Here's how the part is built. I have some questions about the finished solid (model axes, mm). Give positions to 0.01 mm unless a question says otherwise; leave off trailing zeros. Loops run counter-clockwise (first coordinate to the right, second up) from the corner with the lowest first, then second, coordinate; pieces in that order, holes last. Notation, with made-up numbers: (13, 84) - (60, 84) arc R17 cw to (60, 90) - close; hole circle Ø9 at (27, 42.25). An arc over 180 degrees is marked (long way). Use one line per item in the form item = value.
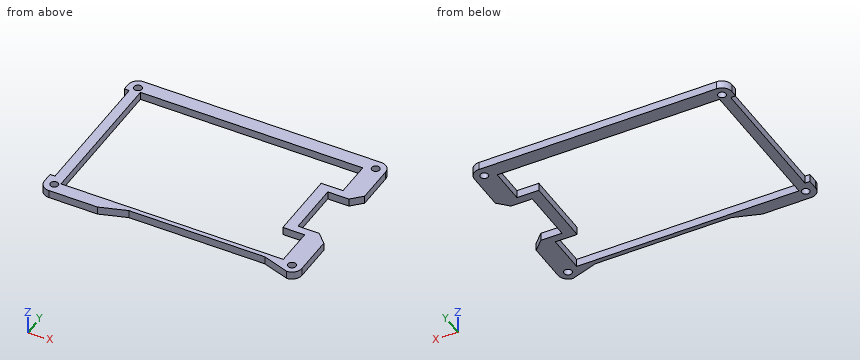
from build123d import *

# Parameters (mm, degrees)
BOSS_EXTRUDE1_DEPTH = 3.048
SKETCH2_R           = 1.355900406
CUT_EXTRUDE1_DEPTH  = 430.898988368
SKETCH3_R           = 1.524
CUT_EXTRUDE2_DEPTH  = 430.898988368
CUT_EXTRUDE3_DEPTH  = 430.898988368
SKETCH4_4_W         = 8.3947
SKETCH4_4_H         = 2.41935
BOSS_EXTRUDE2_DEPTH = 3.048


with BuildPart() as part:
    # Sketch1 → Boss-Extrude1 (new body)
    with BuildSketch(Plane.XY):
        with BuildLine():
            Line((-309.8086, 128.8851), (-305.87795, 128.8851))
            Line((-305.87795, 128.8851), (-301.9473, 132.81575))
            Line((-301.9473, 132.81575), (-301.9473, 150.9704))
            ThreePointArc((-301.9473, 150.9704), (-303.063223164, 153.664476836), (-305.7573, 154.7804))
            Line((-305.7573, 154.7804), (-397.247125, 154.7804))
            ThreePointArc((-397.247125, 154.7804), (-399.946077222, 153.659592612), (-401.0571, 150.956597849))
            Line((-401.0571, 150.956597849), (-401.0571, 148.341))
            Line((-401.0571, 148.341), (-399.1521, 148.341))
            Line((-399.1521, 148.341), (-399.1521, 95.6449))
            Line((-399.1521, 95.6449), (-401.0571, 95.6449))
            Line((-401.0571, 95.6449), (-401.0571, 91.659304166))
            ThreePointArc((-401.0571, 91.659304166), (-399.951018769, 88.947400452), (-397.2472, 87.8217))
            Line((-397.2472, 87.8217), (-378.5565, 87.8217))
            Line((-378.5565, 87.8217), (-368.3165, 91.1883))
            Line((-368.3165, 91.1883), (-315.9973, 91.1883))
            Line((-315.9973, 91.1883), (-305.7573, 87.8217))
            ThreePointArc((-305.7573, 87.8217), (-303.063223164, 88.937623164), (-301.9473, 91.6317))
            Line((-301.9473, 91.6317), (-301.9473, 111.74645))
            Line((-301.9473, 111.74645), (-305.87795, 115.6771))
            Line((-305.87795, 115.6771), (-309.8086, 115.6771))
            Line((-309.8086, 115.6771), (-314.0123, 115.6771))
            Line((-314.0123, 115.6771), (-314.0123, 128.8851))
            Line((-314.0123, 128.8851), (-309.8086, 128.8851))
        make_face()
        Polygon((-395.3675, 92.9525), (-395.3675, 149.2432), (-309.8086, 149.2432), (-309.8086, 132.81575), (-318.2033, 132.81575), (-318.2033, 111.74645), (-309.8086, 111.74645), (-309.8086, 92.9525), align=None, mode=Mode.SUBTRACT)
    extrude(amount=BOSS_EXTRUDE1_DEPTH)

    # Sketch2 → Cut-Extrude1 (cut, through all)
    with BuildSketch(Plane(origin=(0, 0, 0), x_dir=(-1, 0, 0), z_dir=(0, 0, -1))):
        with Locations((305.7573, 150.9704)):
            Circle(SKETCH2_R)
        with Locations((397.247125, 150.9704)):
            Circle(SKETCH2_R)
        with Locations((397.2472, 91.6317)):
            Circle(SKETCH2_R)
        with Locations((305.7573, 91.6317)):
            Circle(SKETCH2_R)
    extrude(amount=-CUT_EXTRUDE1_DEPTH, mode=Mode.SUBTRACT)

    # Sketch3 → Cut-Extrude2 (cut, through all)
    with BuildSketch(Plane(origin=(0, 0, 0), x_dir=(-1, 0, 0), z_dir=(0, 0, -1))):
        with Locations((305.7573, 150.9704)):
            Circle(SKETCH3_R)
        with Locations((397.247125, 150.9704)):
            Circle(SKETCH3_R)
        with Locations((397.2472, 91.6317)):
            Circle(SKETCH3_R)
        with Locations((305.7573, 91.6317)):
            Circle(SKETCH3_R)
    extrude(amount=-CUT_EXTRUDE2_DEPTH, mode=Mode.SUBTRACT)

    # Sketch4 → Cut-Extrude3 (cut, through all)
    with BuildSketch(Plane.XY.offset(3.048)):
        Polygon((-301.9473, 111.74645), (-301.9473, 132.81575), (-305.87795, 128.8851), (-314.0123, 128.8851), (-314.0123, 115.6771), (-305.87795, 115.6771), align=None)
        Polygon((-301.9473, 132.81575), (-301.9473, 136.11775), (-305.87795, 132.1871), (-314.0123, 132.1871), (-314.0123, 128.8851), (-305.87795, 128.8851), align=None)
        Polygon((-301.9473, 107.17445), (-301.9473, 111.74645), (-305.87795, 115.6771), (-314.0123, 115.6771), (-314.0123, 111.74645), (-309.8086, 111.74645), (-309.8086, 111.1051), (-305.87795, 111.1051), align=None)
    extrude(amount=-CUT_EXTRUDE3_DEPTH, mode=Mode.SUBTRACT)

    # Sketch4<4> → Boss-Extrude2 (add)
    with BuildSketch(Plane.XY.offset(3.048)):
        Polygon((-301.9473, 104.12645), (-301.9473, 107.17445), (-305.87795, 111.1051), (-309.8086, 111.1051), (-309.8086, 108.0571), (-305.87795, 108.0571), align=None)
        Polygon((-314.0123, 111.1051), (-314.0123, 111.74645), (-318.2033, 111.74645), (-318.2033, 108.0571), (-309.8086, 108.0571), (-309.8086, 111.1051), align=None)
        with Locations((-314.00595, 134.025425)):
            Rectangle(SKETCH4_4_W, SKETCH4_4_H)
    extrude(amount=-BOSS_EXTRUDE2_DEPTH)


solid = part.part
(1) If we section it at C-C (y = 105): List the corners of the cut face in (x, z) for me, plus the area to 3 significant figures.
Geometry says:
outline = (-399.15, 0) - (-395.37, 0) - (-395.37, 3.05) - (-399.15, 3.05) - close; (-309.81, 0) - (-301.95, 0) - (-301.95, 3.05) - (-309.81, 3.05) - close
area = 35.5 mm²
(2) If I drill on probe 1 along X at (y, z) = (151, 1.5); probe 2 along X at (y, z) = (95, 1.35); probe 3 along Y at (x, z) = (-318.5, 0.3), over which ranges is the centre line in solid material (lowest first)?
Geometry says:
probe_1 = -401.06 to -398.77, -395.72 to -307.28, -304.23 to -301.95
probe_2 = -401.06 to -395.37, -309.81 to -301.95
probe_3 = 91.19 to 92.95, 149.24 to 154.78
(3) If we section it at B-B (z = 0.6): Give the number of separate pieces and of enclosed holes in the cut face, plus the area to 3 significant figures.
Geometry says:
separate_pieces = 1
enclosed_holes = 5
area = 1,430 mm²
(4) If we section it at A-A (x = -336): List the corners of the cut face in (y, z) for me, plus the area to 3 significant figures.
Geometry says:
outline = (91.19, 0) - (92.95, 0) - (92.95, 3.05) - (91.19, 3.05) - close; (149.24, 0) - (154.78, 0) - (154.78, 3.05) - (149.24, 3.05) - close
area = 22.3 mm²
(5) For P1, Ø0.6, axis at x = -400.5, z = 1, coming from the -Y side; P2, Ø1.5, axis at y = 119.5, z = 2.5, coming from the -X side; P3, Ø1.8, axis at x = -305.76, y = 91.63, coming from the +Z side; P4, Ø0.6, axis at x = -400.5, z = 1.5, coming from the +Y side, each with a flat end and sliding along its axis, tell me the tip position at first contact or that it passes through.
Geometry says:
P1 = 89.22
P2 = -399.15
P3 = through
P4 = 153.38
